from build123d import *

# Parameters (mm, degrees)
F0_R     = 2.4534575641
F1_DEPTH = 25.4


with BuildPart() as f1:
    # F0 (on Front) → F1 (new body)
    with BuildSketch(Plane.XZ):
        with BuildLine():
            ThreePointArc((-9.5217293486, 51.0495900878), (-6.822864889, 44.1536371069), (0, 41.275))
            ThreePointArc((0, 41.275), (6.7351920908, 44.0648079092), (9.525, 50.8))
            ThreePointArc((9.525, 50.8), (0.1248057582, 60.3241823021), (-9.5217293486, 51.0495900878))
        make_face()
        with BuildLine():
            ThreePointArc((3.175, 50.8), (2.2450640303, 48.5549359697), (0, 47.625))
            ThreePointArc((0, 47.625), (-2.2450640303, 53.0450640303), (3.175, 50.8))
        make_face(mode=Mode.SUBTRACT)
        with BuildLine():
            ThreePointArc((9.525, 50.8), (6.7351920908, 44.0648079092), (0, 41.275))
            Line((0, 41.275), (0, 15.875))
            ThreePointArc((0, 15.875), (10.4912828764, 11.9142187578), (15.747456912, 2.0082892734))
            Line((15.747456912, 2.0082892734), (9.525, 50.8))
        make_face()
        with BuildLine():
            Line((0, 15.875), (0, 41.275))
            ThreePointArc((0, 41.275), (-6.822864889, 44.1536371069), (-9.5217293486, 51.0495900878))
            Line((-9.5217293486, 51.0495900878), (-15.74860511, 1.9992653877))
            ThreePointArc((-15.74860511, 1.9992653877), (-10.4946959692, 11.9112124284), (0, 15.875))
        make_face()
        with Locations((-3.8164881989, 36.5252)):
            Circle(F0_R, mode=Mode.SUBTRACT)
        with BuildLine():
            ThreePointArc((15.747456912, 2.0082892734), (10.4912828764, 11.9142187578), (0, 15.875))
            Line((0, 15.875), (0, 3.175))
            ThreePointArc((0, 3.175), (2.2450640303, 2.2450640303), (3.175, 0))
            ThreePointArc((3.175, 0), (2.2450640303, -2.2450640303), (0, -3.175))
            Line((0, -3.175), (0, -15.875))
            ThreePointArc((0, -15.875), (11.2253201513, -11.2253201513), (15.875, 0))
            ThreePointArc((15.875, 0), (15.8430821414, 1.0061676109), (15.747456912, 2.0082892734))
        make_face()
        with BuildLine():
            Line((0, 3.175), (0, 15.875))
            ThreePointArc((0, 15.875), (-10.4946959692, 11.9112124284), (-15.74860511, 1.9992653877))
            ThreePointArc((-15.74860511, 1.9992653877), (-11.9112124284, -10.4946959692), (0, -15.875))
            Line((0, -15.875), (0, -3.175))
            ThreePointArc((0, -3.175), (-3.175, 0), (0, 3.175))
        make_face()
        with BuildLine():
            Line((16.0035761028, 0), (15.747456912, 2.0082892734))
            ThreePointArc((15.747456912, 2.0082892734), (15.8430821414, 1.0061676109), (15.875, 0))
            ThreePointArc((15.875, 0), (11.2253201513, -11.2253201513), (0, -15.875))
            Line((0, -15.875), (0, -53.975))
            ThreePointArc((0, -53.975), (6.7351920908, -56.7648079092), (9.525, -63.5))
            Line((9.525, -63.5), (36.5125, -63.5))
            ThreePointArc((36.5125, -63.5), (38.9380895153, -57.7883672161), (44.7324052746, -55.5675253854))
            Line((44.7324052746, -55.5675253854), (18.9822637558, -54.6507905531))
            ThreePointArc((18.9822637558, -54.6507905531), (13.2731893708, -51.9307973584), (11.3553673773, -45.9046997726))
            Line((11.3553673773, -45.9046997726), (16.0035761028, 0))
        make_face()
        with BuildLine():
            ThreePointArc((0, -15.875), (-11.9112124284, -10.4946959692), (-15.74860511, 1.9992653877))
            Line((-15.74860511, 1.9992653877), (-16.0024092847, 0))
            Line((-16.0024092847, 0), (-9.4765589271, -64.4594039301))
            ThreePointArc((-9.4765589271, -64.4594039301), (-7.0662559901, -57.1130092154), (0, -53.975))
            Line((0, -53.975), (0, -15.875))
        make_face()
        with BuildLine():
            Line((0, -60.325), (0, -53.975))
            ThreePointArc((0, -53.975), (-7.0662559901, -57.1130092154), (-9.4765589271, -64.4594039301))
            ThreePointArc((-9.4765589271, -64.4594039301), (-6.3869907846, -70.5662559901), (0, -73.025))
            Line((0, -73.025), (0.6773435479, -73.000885786))
            ThreePointArc((0.6773435479, -73.000885786), (6.9705567315, -69.9912990883), (9.525, -63.5))
            Line((9.525, -63.5), (3.175, -63.5))
            ThreePointArc((3.175, -63.5), (-2.2450640303, -65.7450640303), (0, -60.325))
        make_face()
        with BuildLine():
            Line((36.5125, -63.5), (9.525, -63.5))
            ThreePointArc((9.525, -63.5), (6.9705567315, -69.9912990883), (0.6773435479, -73.000885786))
            Line((0.6773435479, -73.000885786), (44.7324052746, -71.4324746146))
            ThreePointArc((44.7324052746, -71.4324746146), (38.9380895153, -69.2116327839), (36.5125, -63.5))
        make_face()
        with BuildLine():
            Line((0.6773435479, -73.000885786), (0, -73.025))
            ThreePointArc((0, -73.025), (0.3388863295, -73.0189695375), (0.6773435479, -73.000885786))
        make_face()
        with BuildLine():
            ThreePointArc((52.3875, -63.5), (50.1616327839, -57.9880895153), (44.7324052746, -55.5675253854))
            ThreePointArc((44.7324052746, -55.5675253854), (38.9380895153, -57.7883672161), (36.5125, -63.5))
            ThreePointArc((36.5125, -63.5), (38.9380895153, -69.2116327839), (44.7324052746, -71.4324746146))
            ThreePointArc((44.7324052746, -71.4324746146), (50.1616327839, -69.0119104847), (52.3875, -63.5))
        make_face()
        with BuildLine():
            ThreePointArc((47.625, -63.5), (44.45, -66.675), (41.275, -63.5))
            ThreePointArc((41.275, -63.5), (44.45, -60.325), (47.625, -63.5))
        make_face(mode=Mode.SUBTRACT)
        with BuildLine():
            ThreePointArc((9.525, -63.5), (6.7351920908, -56.7648079092), (0, -53.975))
            Line((0, -53.975), (0, -60.325))
            ThreePointArc((0, -60.325), (2.2450640303, -61.2549359697), (3.175, -63.5))
            Line((3.175, -63.5), (9.525, -63.5))
        make_face()
    extrude(amount=F1_DEPTH)


solid = f1.part
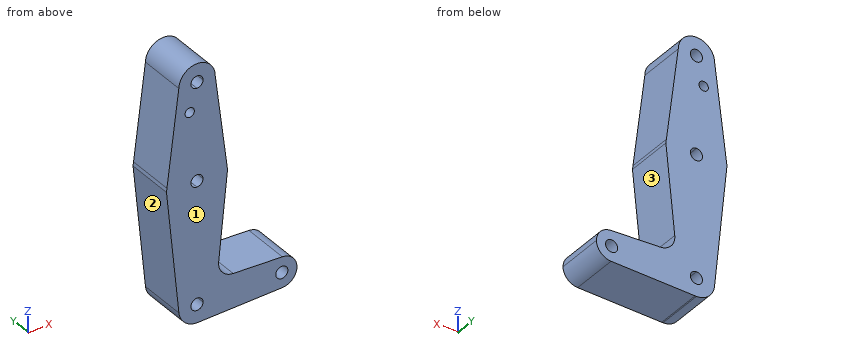
Can you work these out from the model? Positions are in its coordinate system, mm. Face numbers are marked on the shaded views. Give positions to 0.01 mm unless a question says otherwise; leave off trailing zeros. Loops run counter-clockwise (first coordinate to the right, second up) from the corner with the lowest first, then second, coordinate; pieces in that order, holes last. Notation, with made-up numbers: (73, 55) -> (127, 55) arc R22 cw to (127, 66) -> close; hole circle Ø2 at (39, 45.5). An arc over 180 degrees is marked (long way). Return JSON: item names as keys, results as strings.
Q1. We'd pull the mould along Z, two halves only. Please class the marked faces 1, 2 and 3: released by +Z, released by -Z, zero draft, split by the parting line, or undercut.
Checks:
{"face 1": "zero draft", "face 2": "released by -Z", "face 3": "undercut"}
Q2. I want a section at C-C, the plane z = 43.5. List the corners of the cut face in (x, y) for me.
Checks:
{"outline": "(-10.48, -25.4) -> (10.46, -25.4) -> (10.46, 0) -> (-10.48, 0) -> close"}
Q3. I want a section at A-A, the plane y = -8. Count the separate pieces of the cut face and the enclosed holes in it, then the cut area to 3 significant figures.
Checks:
{"separate pieces": "1", "enclosed holes": "5", "area": "3,790 mm2"}
Q4. I need wall thicknesses on probe 1 along Z at (x, y) = (44.45, -9.5) (3 decimals); probe 2 along X at (y, z) = (-16.5, -63.5) (1 decimal); probe 3 along X at (y, z) = (-20.5, 37). Which ranges of each line are inside material? Lowest first, please.
Checks:
{"probe 1": "z = -71.443 to -66.675, -60.325 to -55.557", "probe 2": "x = -9.6 to -3.2, 3.2 to 41.3, 47.6 to 52.4", "probe 3": "x = -11.31 to -6.22, -1.41 to 11.28"}
Q5. I want a section at B-B, the plane z = -32.5. List the corners of the cut face in (x, y) for me.
Checks:
{"outline": "(-12.71, -25.4) -> (12.71, -25.4) -> (12.71, 0) -> (-12.71, 0) -> close"}
Q6. For pin 1 Ø5 at (x, y) = (43.5, -5.5) entering from -Z; pin 2 Ø8 at (x, y) = (12, -2.5) entering from +Z; pin 3 Ø5 at (x, y) = (32.5, -4) entering from -Z; pin 4 Ø5.5 at (x, z) = (44.45, -63.5) entering from -Y, each with a flat end and sliding along its axis, tell me the tip position at first contact or that it passes through.
Checks:
{"pin 1": "stops at z = -71.57", "pin 2": "stops at z = 55.97", "pin 3": "stops at z = -71.96", "pin 4": "passes through"}
